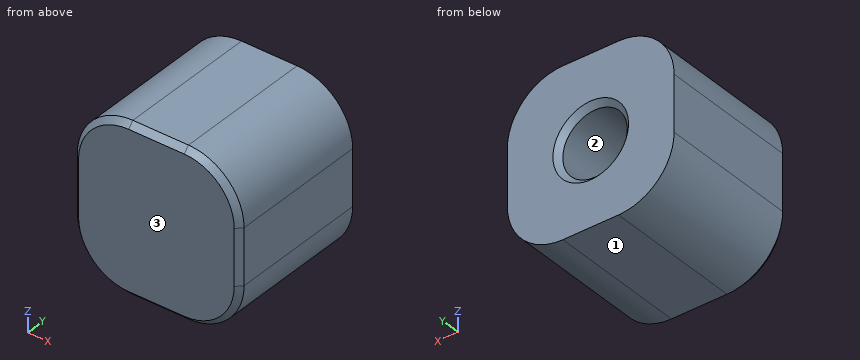
```python
from build123d import *

# Parameters (mm, degrees)
SKETCH_1_W          = 30
SKETCH_1_H          = 30
EXTRUDE_1_DEPTH     = 26
SKETCH_2_R          = 5.8
CUT_EXTRUDE_1_DEPTH = 20
FILLET_1_R          = 10
CHAMFER_1_SIZE      = 1
CHAMFER_2_SIZE      = 1


with BuildPart() as part:
    # Эскиз1 → Бобышка-Вытянуть1 (new body)
    with BuildSketch(Plane(origin=(0, 0, 0), x_dir=(1, 0, 0), z_dir=(0, 1, 0))):
        Rectangle(SKETCH_1_W, SKETCH_1_H)
    extrude(amount=EXTRUDE_1_DEPTH)

    # Эскиз2 → Вырез-Вытянуть1 (cut)
    with BuildSketch(Plane(origin=(0, 26, 0), x_dir=(1, 0, 0), z_dir=(0, 1, 0))):
        with Locations(Location((0, 0, 0), (0, 0, 270))):
            Circle(SKETCH_2_R)
    extrude(amount=-CUT_EXTRUDE_1_DEPTH, mode=Mode.SUBTRACT)

    # Скругление1
    fillet_1_edges = [part.edges().sort_by_distance(p)[0] for p in [
        (15, 13, 15),
        (-15, 13, 15),
        (-15, 13, -15),
        (15, 13, -15),
    ]]
    fillet(fillet_1_edges, radius=FILLET_1_R)

    # Фаска1
    chamfer_1_edges = [part.edges().sort_by_distance(p)[0] for p in [
        (-15, 0, 0),
        (15, 0, 0),
        (0, 0, 15),
        (0, 0, -15),
        (12.071067812, 0, 12.071067812),
        (-12.071067812, 0, 12.071067812),
        (12.071067812, 0, -12.071067812),
        (-12.071067812, 0, -12.071067812),
    ]]
    chamfer(chamfer_1_edges, length=CHAMFER_1_SIZE)

    # Фаска2
    chamfer_2_edges = [part.edges().sort_by_distance(p)[0] for p in [
        (0, 26, -5.8),
    ]]
    chamfer(chamfer_2_edges, length=CHAMFER_2_SIZE)


solid = part.part
```
Part model, mm, in its own coordinate system. Face numbers are marked on the shaded views. Give positions to 0.01 mm unless a question says otherwise; leave off trailing zeros. Order: outer loops, then holes, each group sorted by start corner. A loop starts at its lowest first (then second) coordinate and runs counter-clockwise, first axis right, second up. Notation, with made-up numbers: (30, 15.5) - (51, 15.5) arc R25 ccw to (51, 52.5) - close; hole circle Ø9 at (20.5, -20.5). An arc over 180 degrees is marked (long way). Use one line per item in the form item = value.
Item 1: Pin check, flat tips, straight feed: pin 1 Ø3 at (y, z) = (22, 11) entering from +X; pin 2 Ø5 at (x, y) = (-10.5, 23.5) entering from -Z; pin 3 Ø10.5 at (x, z) = (0, 0) entering from +Y. Stop position of each tip, or through.
Solution:
pin_1 = 13.93
pin_2 = -14.54
pin_3 = 6
Item 2: Slice it at C-C on x = 0. Give the cut face in (y, z), and give its area (3 significant figures).
Solution:
outline = (0, -14) - (1, -15) - (26, -15) - (26, -6.8) - (25, -5.8) - (6, -5.8) - (6, 5.8) - (25, 5.8) - (26, 6.8) - (26, 15) - (1, 15) - (0, 14) - close
area = 546 mm2
Item 3: Slice it at A-A on y = 8.25. Give the cut face in (x, z), and give its area (3 significant figures).
Solution:
outline = (-15, -5) arc R10 ccw to (-5, -15) - (5, -15) arc R10 ccw to (15, -5) - (15, 5) arc R10 ccw to (5, 15) - (-5, 15) arc R10 ccw to (-15, 5) - close; hole circle Ø11.6 at (0, 0)
area = 708 mm2
Item 4: Two-plate mould, pull along Z, no slides. Class the marked faces 1, 2 and 3: released by +Z, released by -Z, zero draft, split by the parting line, or undercut.
Solution:
face_1 = released by -Z
face_2 = undercut
face_3 = zero draft
Item 5: Probe probe 1 along X at (y, z) = (20, 0); probe 2 along X at (y, z) = (21.25, -3); probe 3 along Z at (x, y) = (-5, 19.25). List the from-to ranges inside material, lowest first. Write a range as from..to.
Solution:
probe_1 = -15..-5.8, 5.8..15
probe_2 = -15..-4.96, 4.96..15
probe_3 = -15..-2.94, 2.94..15
Item 6: Slice it at B-B on z = 0. Give the cut face in (x, y), and give its area (3 significant figures).
Solution:
outline = (-15, 1) - (-14, 0) - (14, 0) - (15, 1) - (15, 26) - (6.8, 26) - (5.8, 25) - (5.8, 6) - (-5.8, 6) - (-5.8, 25) - (-6.8, 26) - (-15, 26) - close
area = 546 mm2
